Autodesk Inventor part; units mm, degrees
ref_plane "YZ Plane" through (0, 0, 0) normal (1, 0, 0) x (0, 1, 0)
ref_plane "XZ Plane" through (0, 0, 0) normal (0, 1, 0) x (-1, 0, 0)
ref_plane "XY Plane" through (0, 0, 0) normal (0, 0, 1) x (1, 0, 0)
sketch "Sketch1" plane through (0, 0, 0) normal (0, 0, 1) x (1, 0, 0)
  line L0 (15.5, -21.15) -> (-15.5, -21.15)
  line L1 (-21.15, -15.5) -> (-21.15, 15.5)
  line L2 (-15.5, 21.15) -> (15.5, 21.15)
  line L3 (21.15, 15.5) -> (21.15, -15.5)
  line L4 (21.15, -21.15) -> (-21.15, 21.15) construction
  line L5 (-21.15, -21.15) -> (21.15, 21.15) construction
  line L6 (-15.5, 21.15) -> (-21.15, 15.5)
  line L7 (-21.15, 0) -> (-21.15, 15.5)
  line L8 (0, 21.15) -> (-15.5, 21.15)
  line L9 (15.5, 21.15) -> (21.15, 15.5)
  line L10 (21.15, -15.5) -> (15.5, -21.15)
  line L11 (-15.5, -21.15) -> (-21.15, -15.5)
  point P0 (0, 0)
  dimension "d0" = 42.3
  dimension "d1" = 42.3
  dimension "d2" = 5.65
  dimension "d3" = 5.65
  dimension "d4" = 15.5
  dimension "d5" = 15.5
extrude "Extrusion1" add sketch "Sketch1" against normal blind 40
sketch "Sketch2" plane through (0, 0, 0) normal (0, 0, 1) x (1, 0, 0)
  circle A0 centre (0, 0) radius 11
  dimension "d8" = 22
extrude "Extrusion2" add sketch "Sketch2" along normal blind 2
sketch "Sketch3" plane through (0, 0, 0) normal (0, 0, 1) x (1, 0, 0)
  circle A0 centre (0, 0) radius 2.5
  dimension "d11" = 5
extrude "Extrusion3" add sketch "Sketch3" along normal blind 24
chamfer "Chamfer1" distance 0.5 angle 45 1 edges at (-2.5, 0, 24)
sketch "Sketch4" plane through (0, 0, 0) normal (0, 0, 1) x (1, 0, 0)
  line L0 (-21.15, 15.5) -> (-21.15, -15.5)
  line L1 (-15.5, 21.15) -> (-21.15, 15.5)
  circle A0 centre (-15.1766, 15.5) radius 1.5
  circle A1 centre (15.5, 15.5) radius 1.5
  circle A2 centre (-15.5, -15.5) radius 1.5
  circle A3 centre (15.5, -15.5) radius 1.5
  point P0 (0, 0)
  dimension "d18" = 3
  dimension "d19" = 3
  dimension "d20" = 3
  dimension "d21" = 3
extrude "Extrusion4" cut sketch "Sketch4" against normal blind 4.5
sketch "Sketch5" plane through (-15.5, -21.15, 0) normal (0, -1, 0) x (1, 0, 0)
  point P0 (15.5, 0)
sketch "Sketch6" plane through (21.15, -15.5, 0) normal (1, 0, 0) x (0, 0, -1)
  line L0 (40, 0) -> (40, 31)
  line L1 (38, 11.5) -> (34, 11.5)
  line L2 (34, 11.5) -> (34, 19.5)
  line L3 (34, 19.5) -> (38, 19.5)
  line L4 (38, 19.5) -> (38, 11.5)
  line L5 (38, 11.5) -> (34, 19.5) construction
  line L6 (34, 11.5) -> (38, 19.5) construction
  line L7 (0, 0) -> (40, 0)
  line L8 (0, 31) -> (40, 31)
  point P0 (0, 15.5)
  point P1 (40, 15.5)
  point P2 (36, 15.5)
  dimension "d24" = 4
  dimension "d25" = 8
  dimension "d26" = 2
  dimension "d29" = 15.5
  dimension "d30" = 31
extrude "Extrusion5" add sketch "Sketch6" along normal blind 2
equation "\"d3\" = d2"
properties part number "Motor BYGHW609"
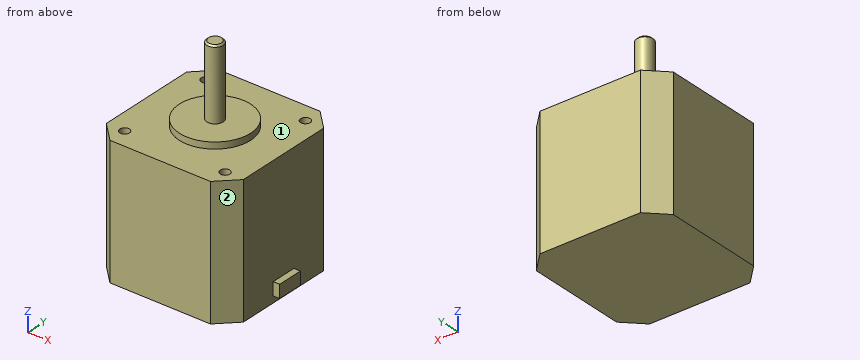
The listing builds one solid part. Answer for the finished solid, in the listing's coordinates (mm). Face numbers are marked on the shaded views. A direction names the side the tool comes from. Coordinates: 2 decimals unless noted, no trailing zeros. Loops run counter-clockwise (first coordinate to the right, second up) from the corner with the lowest first, then second, coordinate; pieces in that order, holes last. Notation, with made-up numbers: (60.25, 78.5) - (114.25, 78.5) arc R12 ccw to (114.25, 84.5) - close; hole circle Ø4 at (62.25, -19). An arc over 180 degrees is marked (long way). Use a Markdown table: item, result. Add a question column.
1) Given pin 1 (2 mm diameter, centred on x = 22.5, y = -0.5, fed in from +Z); pin 2 (0.6 mm diameter, centred on x = 22.5, z = -36, fed in from +Y); pin 3 (2.5 mm diameter, centred on x = 15.5, y = -15.5, fed in from +Z), each flat-ended and moving along its own axis, determine where each tip first touches the part or whether it passes through.
2) The part is cut by section C-C, the plane z = -22. Give the vertices of the cut face in (x, y), and give its area (3 significant figures).
3) The part is cut by section B-B, the plane y = 0. Give the vertices of the cut face in (x, z).
4) The part is cut by section D-D, the plane y = 18.5. Give the vertices of the cut face in (x, z).
5) The part is cut by section A-A, the plane x = 0. Give the vertices of the cut face in (y, z), and give its area (3 significant figures).
6) For the marked faces 1 and 2, determine the directions among +Z, -Z, +X, -X, +Y, -Y from which every point of the face is accessible in a straight line to the end or side of a thin tool.
7) Find the intervals of material crossed by line 1 (X direction, y = -15, z = -1); line 2 (X direction, y = 15, z = -2); line 3 (Z direction, x = 7.5, y = -11), in increasing order.
Here are the results:
| question | item | result |
|---|---|---|
| 1 | pin 1 | stops at z = -34 |
| 1 | pin 2 | stops at y = 4 |
| 1 | pin 3 | stops at z = -4.5 |
| 2 | outline | (-21.15, -15.5) - (-15.5, -21.15) - (15.5, -21.15) - (21.15, -15.5) - (21.15, 15.5) - (15.5, 21.15) - (-15.5, 21.15) - (-21.15, 15.5) - close |
| 2 | area | 1,730 mm^2 |
| 3 | outline | (-21.15, -40) - (21.15, -40) - (21.15, -38) - (23.15, -38) - (23.15, -34) - (21.15, -34) - (21.15, 0) - (11, 0) - (11, 2) - (2.5, 2) - (2.5, 23.5) - (2, 24) - (-2, 24) - (-2.5, 23.5) - (-2.5, 2) - (-11, 2) - (-11, 0) - (-21.15, 0) - close |
| 4 | outline | (-18.15, -40) - (18.15, -40) - (18.15, 0) - (-18.15, 0) - close |
| 5 | outline | (-21.15, -40) - (21.15, -40) - (21.15, 0) - (11, 0) - (11, 2) - (2.5, 2) - (2.5, 23.5) - (2, 24) - (-2, 24) - (-2.5, 23.5) - (-2.5, 2) - (-11, 2) - (-11, 0) - (-21.15, 0) - close |
| 5 | area | 1,850 mm^2 |
| 6 | face 1 | +Z |
| 6 | face 2 | +Z, -Z, +X, -Y |
| 7 | line 1 | x = -21.15 to -16.91, -14.09 to 14.09, 16.91 to 21.15 |
| 7 | line 2 | x = -21.15 to -16.59, -13.76 to 14.09, 16.91 to 21.15 |
| 7 | line 3 | z = -40 to 0 |
